Build history of the part. All positions in model axes, mm. Face numbers are marked on the shaded views. A direction names the side the tool comes from. Give positions to 0.01 mm unless a question says otherwise; leave off trailing zeros. Write each loop counter-clockwise with the first axis right and the second up, starting at its lowest first coordinate (ties: lowest second). Pieces come first, ordered by that corner, then holes.
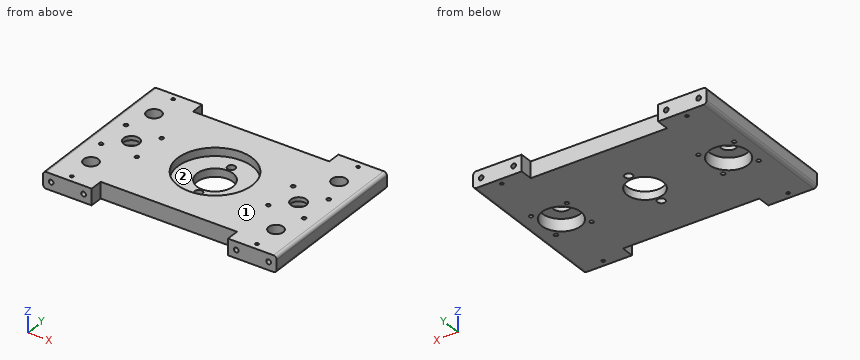
from build123d import *

# Parameters (mm, degrees)
CYLINDER028_R       = 4.8
CYLINDER028_DEPTH   = 10
CYLINDER016_R       = 1.2
CYLINDER016_DEPTH   = 20
ARRAY001006_X_COUNT = 2
ARRAY001006_X_PITCH = 22
ARRAY001006_Y_COUNT = 2
ARRAY001006_Y_PITCH = 22
CYLINDER026_R       = 12
CYLINDER026_DEPTH   = 10
CYLINDER027_R       = 4.5
CYLINDER027_DEPTH   = 24
ARRAY001008_Y_COUNT = 2
ARRAY001008_Y_PITCH = 56
CYLINDER040_R       = 1
CYLINDER040_DEPTH   = 20
ARRAY001022_Y_COUNT = 2
ARRAY001022_Y_PITCH = 90
CYLINDER039_R       = 1.45
CYLINDER039_DEPTH   = 40
ARRAY001020_X_COUNT = 2
ARRAY001020_X_PITCH = 20
ARRAY001020_Y_COUNT = 2
ARRAY001020_Y_PITCH = 80
CYLINDER037_R       = 23
CYLINDER037_DEPTH   = 30
CYLINDER036_R       = 2.4
CYLINDER036_DEPTH   = 30
ARRAY001018_Y_COUNT = 2
ARRAY001018_Y_PITCH = 29
CYLINDER029_R       = 11.1
CYLINDER029_DEPTH   = 30
BOX004_W            = 144
BOX004_H            = 82
BOX004_DEPTH        = 10
BOX019_W            = 30
BOX019_H            = 98
BOX019_DEPTH        = 10
FILLET004_R         = 2


with BuildPart() as bottom_side_lead_hole:
    # Cylinder028 → Cylinder028 (new body)
    with BuildSketch(Plane.XY.offset(4)):
        Circle(CYLINDER028_R)
    extrude(amount=CYLINDER028_DEPTH)


with BuildPart() as lead_holder_hole_array:
    # Cylinder016 → Cylinder016 (new body)
    with BuildSketch(Plane(origin=(-11, -11, 0), x_dir=(1, 0, 0), z_dir=(0, 0, 1))):
        Circle(CYLINDER016_R)
    extrude(amount=CYLINDER016_DEPTH)

    # Array001006 X: lead holder hole array ×2


with BuildPart() as lead_holder_hole_array_1:
    add(lead_holder_hole_array.part)
    with Locations(*[(i * ARRAY001006_X_PITCH, 0, 0) for i in range(1, ARRAY001006_X_COUNT)]):
        add(lead_holder_hole_array.part)

    # Array001006 Y: lead holder hole array ×2


with BuildPart() as lead_holder_hole_array_2:
    add(lead_holder_hole_array_1.part)
    with Locations(*[(0, i * ARRAY001006_Y_PITCH, 0) for i in range(1, ARRAY001006_Y_COUNT)]):
        add(lead_holder_hole_array_1.part)


with BuildPart() as lead_holder_hole_array_3:
    # Array001006 placement: moved
    add(lead_holder_hole_array_2.part.moved(Location((0, 0, -5))))


with BuildPart() as lead_bottom_hole_fusion:
    # Cylinder026 → Cylinder026 (new body)
    with BuildSketch(Plane.XY.offset(-2.5)):
        Circle(CYLINDER026_R)
    extrude(amount=CYLINDER026_DEPTH)

    # Fusion029: union bottom side lead hole, lead holder hole array
    add(bottom_side_lead_hole.part)
    add(lead_holder_hole_array_3.part)


with BuildPart() as lead_bottom_hole_fusion_1:
    # Fusion029 placement: moved
    add(lead_bottom_hole_fusion.part.moved(Location((20.5, 41, 0))))


with BuildPart() as rod_holder_hole_array_array:
    # Cylinder027 → Cylinder027 (new body)
    with BuildSketch(Plane.XY.offset(3)):
        Circle(CYLINDER027_R)
    extrude(amount=CYLINDER027_DEPTH)

    # Array001008 Y: rod holder hole array array ×2


with BuildPart() as rod_holder_hole_array_array_1:
    add(rod_holder_hole_array_array.part)
    with Locations(*[(0, i * ARRAY001008_Y_PITCH, 0) for i in range(1, ARRAY001008_Y_COUNT)]):
        add(rod_holder_hole_array_array.part)


with BuildPart() as rod_holder_hole_array_array_2:
    # Array001008 placement: moved
    add(rod_holder_hole_array_array_1.part.moved(Location((15, 13, 0))))


with BuildPart() as pusher_hole_array:
    # Cylinder040 → Cylinder040 (new body)
    with BuildSketch(Plane.XY.offset(-5)):
        Circle(CYLINDER040_R)
    extrude(amount=CYLINDER040_DEPTH)

    # Array001022 Y: pusher hole array ×2


with BuildPart() as pusher_hole_array_1:
    add(pusher_hole_array.part)
    with Locations(*[(0, i * ARRAY001022_Y_PITCH, 0) for i in range(1, ARRAY001022_Y_COUNT)]):
        add(pusher_hole_array.part)


with BuildPart() as pusher_hole_array_2:
    # Array001022 placement: moved
    add(pusher_hole_array_1.part.moved(Location((15, -4, 0))))


with BuildPart() as bottom_hole_fusion:
    # Cylinder039 → Cylinder039 (new body)
    with BuildSketch(Plane(origin=(0, 0, 5), x_dir=(1, 0, 0), z_dir=(0, -1, 0))):
        Circle(CYLINDER039_R)
    extrude(amount=CYLINDER039_DEPTH)

    # Array001020 X: bottom hole fusion ×2


with BuildPart() as bottom_hole_fusion_1:
    add(bottom_hole_fusion.part)
    with Locations(*[(i * ARRAY001020_X_PITCH, 0, 0) for i in range(1, ARRAY001020_X_COUNT)]):
        add(bottom_hole_fusion.part)

    # Array001020 Y: bottom hole fusion ×2


with BuildPart() as bottom_hole_fusion_2:
    add(bottom_hole_fusion_1.part)
    with Locations(*[(0, i * ARRAY001020_Y_PITCH, 0) for i in range(1, ARRAY001020_Y_COUNT)]):
        add(bottom_hole_fusion_1.part)


with BuildPart() as bottom_hole_fusion_3:
    # Array001020 placement: moved
    add(bottom_hole_fusion_2.part.moved(Location((0, 20, 0))))


with BuildPart() as bottom_hole_fusion_4:
    # Clone007 placement: moved
    add(bottom_hole_fusion_3.part.moved(Location((0, 7, 0))))


with BuildPart() as bottom_hole_fusion_5:
    # Body007 placement: moved
    add(bottom_hole_fusion_4.part.moved(Location((5, 0, 0))))

    # Fusion012: union lead bottom hole fusion, rod holder hole array array, pusher hole array
    add(lead_bottom_hole_fusion_1.part)
    add(rod_holder_hole_array_array_2.part)
    add(pusher_hole_array_2.part)


with BuildPart() as dc_motor_body_bottom_hole:
    # Cylinder037 → Cylinder037 (new body)
    with BuildSketch(Plane.XY.offset(5)):
        Circle(CYLINDER037_R)
    extrude(amount=CYLINDER037_DEPTH)


with BuildPart() as dc_motor_bolt_hole_array:
    # Cylinder036 → Cylinder036 (new body)
    with BuildSketch(Plane.XY):
        Circle(CYLINDER036_R)
    extrude(amount=CYLINDER036_DEPTH)

    # Array001018 Y: dc motor bolt hole array ×2


with BuildPart() as dc_motor_bolt_hole_array_1:
    add(dc_motor_bolt_hole_array.part)
    with Locations(*[(0, i * ARRAY001018_Y_PITCH, 0) for i in range(1, ARRAY001018_Y_COUNT)]):
        add(dc_motor_bolt_hole_array.part)


with BuildPart() as dc_motor_bolt_hole_array_2:
    # Array001018 placement: moved
    add(dc_motor_bolt_hole_array_1.part.moved(Location((0, -14.5, -6))))


with BuildPart() as dc_motor_bottom_hole_fusion:
    # Cylinder029 → Cylinder029 (new body)
    with BuildSketch(Plane.XY):
        Circle(CYLINDER029_R)
    extrude(amount=CYLINDER029_DEPTH)

    # Fusion028: union dc motor body bottom hole, dc motor bolt hole array
    add(dc_motor_body_bottom_hole.part)
    add(dc_motor_bolt_hole_array_2.part)


with BuildPart() as dc_motor_bottom_hole_fusion_1:
    # Fusion028 placement: moved
    add(dc_motor_bottom_hole_fusion.part.moved(Location((72, 41, 0))))


with BuildPart() as bottom_hole_mirrored_fusion:
    # Part__Mirroring003: instance of bottom hole fusion
    add(bottom_hole_fusion_5.part.mirror(Plane(origin=(72, 0, 0), x_dir=(0, -1, 0), z_dir=(1, 0, 0))))

    # Fusion030: union bottom hole fusion, dc motor bottom hole fusion
    add(bottom_hole_fusion_5.part)
    add(dc_motor_bottom_hole_fusion_1.part)


with BuildPart() as bottom_side_cube:
    # Box004 → Box004 (new body)
    with BuildSketch(Plane.XY):
        with Locations((72, 41)):
            Rectangle(BOX004_W, BOX004_H)
    extrude(amount=BOX004_DEPTH)


with BuildPart() as bottom_side_cube_extension:
    # Box019 → Box019 (new body)
    with BuildSketch(Plane(origin=(0, -8, 0), x_dir=(1, 0, 0), z_dir=(0, 0, 1))):
        with Locations((15, 49)):
            Rectangle(BOX019_W, BOX019_H)
    extrude(amount=BOX019_DEPTH)


with BuildPart() as part_mirroring002:
    # Part__Mirroring002: instance of bottom side cube extension
    add(bottom_side_cube_extension.part.mirror(Plane(origin=(72, 0, 0), x_dir=(0, -1, 0), z_dir=(1, 0, 0))))


with BuildPart() as bottom_side_fillet:
    # Fusion014 base: copy of bottom side cube extension
    add(bottom_side_cube_extension.part)

    # Fusion014: union bottom side cube, Part__Mirroring002
    add(bottom_side_cube.part)
    add(part_mirroring002.part)

    # Cut004: cut bottom hole mirrored fusion
    add(bottom_hole_mirrored_fusion.part, mode=Mode.SUBTRACT)

    # Fillet004
    fillet004_edges = [bottom_side_fillet.edges().sort_by_distance(p)[0] for p in [
        (0, -4, 10),
        (0, -4, 0),
        (0, 41, 10),
        (0, 41, 0),
        (0, 86, 10),
        (0, 86, 0),
        (144, 41, 10),
        (144, 41, 0),
        (144, 86, 10),
        (144, -4, 10),
        (144, -4, 0),
        (144, 86, 0),
    ]]
    fillet(fillet004_edges, radius=FILLET004_R)


solid = bottom_side_fillet.part
1. Saw through at A-A on y = 76.5. Give the cut face in (x, z).
2. Drop flat-ended pins along their axis: pin 1 (2 mm diameter, centred on x = 134.5, y = 30, fed in from -Z); pin 2 (6 mm diameter, centred on x = 54, z = 3.5, fed in from +Y); pin 3 (1.7 mm diameter, centred on x = 25, z = 5, fed in from -Y). Give the stop position or say it passes through.
3. Saw through at B-B on y = 41. Count the separate pieces of the cut face and the enclosed holes in it, plus the area to 3 significant figures.
4. Saw through at C-C on x = 80.5. Give the cut face in (y, z).
5. 3-axis set-ups, long thin cutter, end or side, ignore diameter. For the marked faces 1 and 2: which of +Z, -Z, +X, -X, +Y, -Y reach the whole face in a straight line?
6. Drill centre lines: line 1 along Y through (x, z) = (134.5, 5.25); line 2 along Y through (x, z) = (31.5, 5.25); line 3 along Y through (x, z) = (111.5, 8.75). Where is each one in solid material? Low to high.
7. Saw through at D-D on y = 13. Give the cut face in (x, z).
Outcome:
1. outline: (0, 2) arc R2 ccw to (2, 0) - (142, 0) arc R2 ccw to (144, 2) - (144, 8) arc R2 ccw to (142, 10) - (2, 10) arc R2 ccw to (0, 8) - close; hole circle Ø2.9 at (5, 5); hole circle Ø2.9 at (25, 5); hole circle Ø2.9 at (119, 5); hole circle Ø2.9 at (139, 5)
2. pin 1: passes through
2. pin 2: stops at y = 82
2. pin 3: stops at y = 27
3. separate pieces: 4
3. enclosed holes: 0
3. area: 688 mm2
4. outline: (0, 0) - (33.86, 0) - (33.86, 5) - (19.63, 5) - (19.63, 10) - (0, 10) - close; (48.14, 0) - (82, 0) - (82, 10) - (62.37, 10) - (62.37, 5) - (48.14, 5) - close
5. face 1: +Z, +X, -X, +Y, -Y
5. face 2: +Z
6. line 1: y = -8 to 28.8, 31.2 to 36.2, 45.8 to 50.8, 53.2 to 90
6. line 2: y = 0 to 28.8, 31.2 to 36.2, 45.8 to 50.8, 53.2 to 82
6. line 3: y = 0 to 29.34, 30.66 to 51.34, 52.66 to 82
7. outline: (0, 2) arc R2 ccw to (2, 0) - (142, 0) arc R2 ccw to (144, 2) - (144, 8) arc R2 ccw to (142, 10) - (133.5, 10) - (133.5, 3) - (124.5, 3) - (124.5, 10) - (19.5, 10) - (19.5, 3) - (10.5, 3) - (10.5, 10) - (2, 10) arc R2 ccw to (0, 8) - close; hole circle Ø2.9 at (5, 5); hole circle Ø2.9 at (25, 5); hole circle Ø2.9 at (119, 5); hole circle Ø2.9 at (139, 5)
